Could you check a few things on this model? Use its own coordinates, in mm. Coordinates: 2 decimals unless noted, no trailing zeros. Order: outer loops, then holes, each group sorted by start corner. A loop starts at its lowest first (then second) coordinate and runs counter-clockwise, first axis right, second up. Notation, with made-up numbers: (88, 22) - (124, 22) arc R36 cw to (124, 58) - close; hole circle Ø7 at (-21, 28.5). An arc over 180 degrees is marked (long way). Answer as a JSON object with one key per item and string values. Group by question number.
(1) Imagine slicing it at A-A, the plane y = 0.9. Give the number of separate pieces and of enclosed holes in the cut face, and give its area (3 significant figures).
(2) Imagine slicing it at B-B, the plane x = 12. Write out the boundary of the cut face in (y, z).
(3) Will these pins go through, and if not, where does the flat tip stop? P1, Ø0.5, axis at y = 1, z = 13, coming from the -X side; P2, Ø0.5, axis at x = -4, y = 1, coming from the +Z side; P3, Ø0.5, axis at x = -18.5, y = 0.5, coming from the +Z side.
(4) Imagine slicing it at C-C, the plane z = -14.5. Write out the boundary of the cut face in (x, y).
(5) Please list where these lines run through material, in increasing order: probe 1 along Z at (x, y) = (-113, 0.75); probe 2 along X at (y, z) = (0.1, -9); probe 3 along X at (y, z) = (0.7, -1).
from build123d import *

# Parameters (mm, degrees)
SKETCH_11_W             = 70
SKETCH_11_H             = 12
EXTRUDE_6_DEPTH         = 1.6
SKETCH_12_W             = 3
SKETCH_12_H             = 11.8
CUT_EXTRUDE_6_DEPTH     = 1.6
SKETCH_13_W             = 20
SKETCH_13_H             = 2.2
CUT_EXTRUDE_7_DEPTH     = 1.6
FILLET_1_R              = 1
FILLET_1_OF_MIRROR_15_R = 1
EXTRUDE_7_DEPTH         = 1.6
SKETCH_16_W             = 6
SKETCH_16_H             = 12
EXTRUDE_9_DEPTH         = 1.6
SKETCH_18_W             = 30
SKETCH_18_H             = 49
EXTRUDE_12_DEPTH        = 1.6
FILLET_3_R              = 2
MIRROR_24_OUTLINE_W     = 3
MIRROR_24_OUTLINE_H     = 11.8
MIRROR_24_DEPTH         = 1.6
FILLET_4_R              = 2


# Read off the part's stored shape, not the designer's step: 镜向24
with BuildPart() as part:
    # 草图11 → 凸台-拉伸6 (new body)
    with BuildSketch(Plane(origin=(0, 0, 0), x_dir=(1, 0, 0), z_dir=(0, 1, 0))):
        with Locations((-92.991102456, 0)):
            Rectangle(SKETCH_11_W, SKETCH_11_H)
    extrude(amount=EXTRUDE_6_DEPTH)

    # 草图12 → 切除-拉伸6 (cut)
    with BuildSketch(Plane(origin=(0, 1.6, 0), x_dir=(1, 0, 0), z_dir=(0, 1, 0))):
        with Locations((-69.350034459, 0)):
            Rectangle(SKETCH_12_W, SKETCH_12_H)
    extrude(amount=-CUT_EXTRUDE_6_DEPTH, mode=Mode.SUBTRACT)

    # 草图13 → 切除-拉伸7 (cut)
    with BuildSketch(Plane(origin=(0, 1.6, 0), x_dir=(1, 0, 0), z_dir=(0, 1, 0))):
        with Locations((-112.744310304, 3)):
            Rectangle(SKETCH_13_W, SKETCH_13_H)
    cut_extrude_7 = extrude(amount=-CUT_EXTRUDE_7_DEPTH, mode=Mode.SUBTRACT)

    # 圆角1
    fillet_1_edges = [part.edges().sort_by_distance(p)[0] for p in [
        (-122.744310304, 0.8, -1.9),
        (-122.744310304, 0.8, -4.1),
        (-102.744310304, 0.8, -4.1),
        (-102.744310304, 0.8, -1.9),
    ]]
    fillet(fillet_1_edges, radius=FILLET_1_R)

    # 镜向15: 切除-拉伸7 across plane
    add(cut_extrude_7.mirror(Plane(origin=(0, 0, 0), x_dir=(1, 0, 0), z_dir=(0, 0, -1))), mode=Mode.SUBTRACT)

    # 圆角1 of 镜向15
    fillet_1_of_mirror_15_edges = [part.edges().sort_by_distance(p)[0] for p in [
        (-122.744310304, 0.8, 1.9),
        (-122.744310304, 0.8, 4.1),
        (-102.744310304, 0.8, 4.1),
        (-102.744310304, 0.8, 1.9),
    ]]
    fillet(fillet_1_of_mirror_15_edges, radius=FILLET_1_OF_MIRROR_15_R)

    # 草图14 → 凸台-拉伸7 (add)
    with BuildSketch(Plane(origin=(0, 0, 0), x_dir=(1, 0, 0), z_dir=(0, 1, 0))):
        Polygon((-60.400975616, 6), (-60.400975616, 11.948069584), (-62.610711949, 11.948069584), (-76.405563985, 11.948069584), (-76.405563985, 6), (-74.195827651, 6), (-62.609356584, 6), align=None)
    extrude_7 = extrude(amount=EXTRUDE_7_DEPTH)

    # 镜向17: 凸台-拉伸7 across plane
    add(extrude_7.mirror(Plane(origin=(0, 0, 0), x_dir=(1, 0, 0), z_dir=(0, 0, -1))))

    # 草图16 → 凸台-拉伸9 (add)
    with BuildSketch(Plane(origin=(0, 0, 0), x_dir=(1, 0, 0), z_dir=(0, 1, 0))):
        with Locations((-54.991102456, 0)):
            Rectangle(SKETCH_16_W, SKETCH_16_H)
    extrude(amount=EXTRUDE_9_DEPTH)

    # 草图18 → 凸台-拉伸12 (add)
    with BuildSketch(Plane(origin=(0, 0, 0), x_dir=(1, 0, 0), z_dir=(0, 1, 0))):
        with Locations((-36.991102456, 0)):
            Rectangle(SKETCH_18_W, SKETCH_18_H)
    extrude(amount=EXTRUDE_12_DEPTH)

    # 圆角3
    fillet_3_edges = [part.edges().sort_by_distance(p)[0] for p in [
        (-127.991102456, 0.8, 6),
        (-127.991102456, 0.8, -6),
        (-51.991102456, 0.8, -6),
        (-51.991102456, 0.8, 6),
        (-76.405563985, 0.8, 6),
        (-60.400975616, 0.8, 6),
        (-60.400975616, 0.8, -6),
        (-76.405563985, 0.8, -6),
        (-60.400975616, 0.8, 11.948069584),
        (-76.405563985, 0.8, 11.948069584),
        (-76.405563985, 0.8, -11.948069584),
        (-60.400975616, 0.8, -11.948069584),
    ]]
    fillet(fillet_3_edges, radius=FILLET_3_R)

    # 镜向24 outline → 镜向24 (add)
    with BuildSketch(Plane(origin=(0, 0, 0), x_dir=(1, 0, 0), z_dir=(0, 1, 0))):
        with BuildLine():
            Line((4.423359072, -6), (52.008897544, -6))
            ThreePointArc((52.008897544, -6), (53.423111106, -5.414213562), (54.008897544, -4))
            Line((54.008897544, -4), (54.008897544, 4))
            ThreePointArc((54.008897544, 4), (53.423111106, 5.414213562), (52.008897544, 6))
            Line((52.008897544, 6), (4.423359072, 6))
            ThreePointArc((4.423359072, 6), (3.00914551, 6.585786438), (2.423359072, 8))
            Line((2.423359072, 8), (2.423359072, 9.948069584))
            ThreePointArc((2.423359072, 9.948069584), (1.837572634, 11.362283146), (0.423359072, 11.948069584))
            Line((0.423359072, 11.948069584), (-11.581229297, 11.948069584))
            ThreePointArc((-11.581229297, 11.948069584), (-12.995442859, 11.362283146), (-13.581229297, 9.948069584))
            Line((-13.581229297, 9.948069584), (-13.581229297, 8))
            ThreePointArc((-13.581229297, 8), (-14.167015735, 6.585786438), (-15.581229297, 6))
            Line((-15.581229297, 6), (-19.991102456, 6))
            ThreePointArc((-19.991102456, 6), (-21.405316019, 6.585786437), (-21.991102456, 8))
            Line((-21.991102456, 8), (-21.991102456, -8))
            ThreePointArc((-21.991102456, -8), (-21.405316019, -6.585786437), (-19.991102456, -6))
            Line((-19.991102456, -6), (-15.581229297, -6))
            ThreePointArc((-15.581229297, -6), (-14.167015735, -6.585786438), (-13.581229297, -8))
            Line((-13.581229297, -8), (-13.581229297, -9.948069584))
            ThreePointArc((-13.581229297, -9.948069584), (-12.995442859, -11.362283146), (-11.581229297, -11.948069584))
            Line((-11.581229297, -11.948069584), (0.423359072, -11.948069584))
            ThreePointArc((0.423359072, -11.948069584), (1.837572634, -11.362283146), (2.423359072, -9.948069584))
            Line((2.423359072, -9.948069584), (2.423359072, -8))
            ThreePointArc((2.423359072, -8), (3.00914551, -6.585786438), (4.423359072, -6))
        make_face()
        with Locations((-4.632170453, 0)):
            Rectangle(MIRROR_24_OUTLINE_W, MIRROR_24_OUTLINE_H, mode=Mode.SUBTRACT)
        with BuildLine():
            ThreePointArc((28.762105391, -2.9), (29.05499861, -2.192893219), (29.762105391, -1.9))
            Line((29.762105391, -1.9), (47.762105391, -1.9))
            ThreePointArc((47.762105391, -1.9), (48.469212172, -2.192893219), (48.762105391, -2.9))
            Line((48.762105391, -2.9), (48.762105391, -3.1))
            ThreePointArc((48.762105391, -3.1), (48.469212172, -3.807106781), (47.762105391, -4.1))
            Line((47.762105391, -4.1), (29.762105391, -4.1))
            ThreePointArc((29.762105391, -4.1), (29.05499861, -3.807106781), (28.762105391, -3.1))
            Line((28.762105391, -3.1), (28.762105391, -2.9))
        make_face(mode=Mode.SUBTRACT)
        with BuildLine():
            Line((29.762105391, 4.1), (47.762105391, 4.1))
            ThreePointArc((47.762105391, 4.1), (48.469212172, 3.807106781), (48.762105391, 3.1))
            Line((48.762105391, 3.1), (48.762105391, 2.9))
            ThreePointArc((48.762105391, 2.9), (48.469212172, 2.192893219), (47.762105391, 1.9))
            Line((47.762105391, 1.9), (29.762105391, 1.9))
            ThreePointArc((29.762105391, 1.9), (29.05499861, 2.192893219), (28.762105391, 2.9))
            Line((28.762105391, 2.9), (28.762105391, 3.1))
            ThreePointArc((28.762105391, 3.1), (29.05499861, 3.807106781), (29.762105391, 4.1))
        make_face(mode=Mode.SUBTRACT)
    extrude(amount=MIRROR_24_DEPTH)

    # 圆角4
    fillet_4_edges = [part.edges().sort_by_distance(p)[0] for p in [
        (-21.991102456, 0.8, -24.5),
        (-51.991102456, 0.8, -24.5),
        (-51.991102456, 0.8, 24.5),
        (-21.991102456, 0.8, 24.5),
    ]]
    fillet(fillet_4_edges, radius=FILLET_4_R)


solid = part.part
Result set:
{
 "1": {"separate pieces": "1", "enclosed holes": "6", "area": "3,430 mm^2"},
 "2": {"outline": "(0, -6) - (1.6, -6) - (1.6, 6) - (0, 6) - close"},
 "3": {"P1": "stops at x = -51.99", "P2": "stops at z = 11.95", "P3": "stops at z = 6"},
 "4": {"outline": "(-51.99, 0) - (-21.99, 0) - (-21.99, 1.6) - (-51.99, 1.6) - close"},
 "5": {"probe 1": "z = -6 to -4.1, -1.9 to 1.9, 4.1 to 6", "probe 2": "x = -76.41 to -60.4, -51.99 to -21.99, -13.58 to 2.42", "probe 3": "x = -127.99 to -70.85, -67.85 to -6.13, -3.13 to 54.01"}
}
